The model under review builds one solid part; all positions refer to its coordinate system, in mm. Face numbers are marked on the shaded views. A direction names the side the tool comes from. Round coordinates to 2 decimals unless told otherwise and drop trailing zeros. Order: outer loops, then holes, each group sorted by start corner. A loop starts at its lowest first (then second) coordinate and runs counter-clockwise, first axis right, second up. Notation, with made-up numbers: M 48.5,-13 L 104.5,-13 A29 ccw 104.5,22 Z; hole C 23,22.5 d11. An arc over 180 degrees is marked long. Use a Markdown table: item, result. Add a question column.
1. Consider section D-D on z = -39. State the section outline as (x, y) points.
2. Insertion check: P1, Ø3, axis at x = -26.5, y = 2, coming from the -Z side; P2, Ø4, axis at y = 1.5, z = -83, coming from the -X side; P3, Ø0.8, axis at y = 7, z = -1.5, coming from the -X side; P4, Ø1, axis at x = -2.5, y = 6.5, coming from the -Z side. Each pin has a flat end and moves straight along its axis. Give the tip position at first contact, or say it passes through.
3. Consider section B-B on x = -35.5. State the section outline as (y, z) points, then the cut area to 3 significant figures.
4. For the marked faces 1 and 2, list the 3-axis set-ups (+Z, -Z, +X, -X, +Y, -Y) from which the entire face can be reached by the end or side of a thin tool; tool diameter is ignored.
5. Consider section A-A on z = -6.5. State the section outline as (x, y) points.
6. To check wall thickness, follow probe 1 along X at (y, z) = (4.25, -30); probe 2 along Z at (x, y) = (6, 8.5); probe 3 along Y at (x, z) = (26.5, -9.5). State the ranges of each line that lie inside material, in increasing order.
7. Consider section C-C on y = 7.25. Count the separate pieces of the cut face and the enclosed holes in it, then the cut area to 3 significant figures.
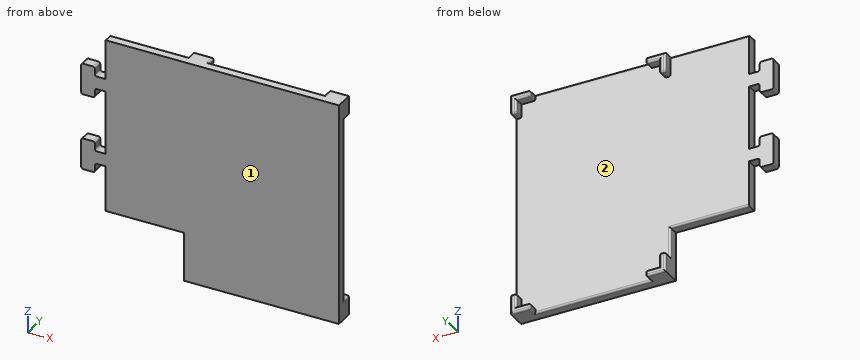
from build123d import *

# Parameters (mm, degrees)
SKETCH1_W           = 79
SKETCH1_H           = 114
BOSS_EXTRUDE1_DEPTH = 5
BOSS_EXTRUDE2_DEPTH = 5
FILLET1_R           = 1
SKETCH3_W           = 89
SKETCH3_H           = 5
BOSS_EXTRUDE3_DEPTH = 40
SKETCH4_W           = 5.5
SKETCH4_H           = 6.5
BOSS_EXTRUDE4_DEPTH = 5
FILLET2_R           = 1
FILLET3_R           = 1


with BuildPart() as part:
    # Sketch1 → Boss-Extrude1 (new body)
    with BuildSketch(Plane(origin=(0, 0, 0), x_dir=(1, 0, 0), z_dir=(0, 1, 0))):
        with Locations((39.5, 57)):
            Rectangle(SKETCH1_W, SKETCH1_H)
    extrude(amount=BOSS_EXTRUDE1_DEPTH)

    # Sketch2 → Boss-Extrude2 (add)
    with BuildSketch(Plane(origin=(0, 5, 0), x_dir=(1, 0, 0), z_dir=(0, 1, 0))):
        Polygon((0, 0), (0, 10), (3, 10), (3, 3), (10, 3), (10, 0), align=None)
        Polygon((79, 0), (69, 0), (69, 3), (76, 3), (76, 10), (79, 10), align=None)
        Polygon((79, 114), (69, 114), (69, 111), (76, 111), (76, 104), (79, 104), align=None)
        Polygon((0, 114), (0, 104), (3, 104), (3, 111), (10, 111), (10, 114), align=None)
    extrude(amount=BOSS_EXTRUDE2_DEPTH)

    # Fillet1
    fillet1_edges = [part.edges().sort_by_distance(p)[0] for p in [
        (10, 7.5, -114),
        (0, 7.5, -104),
        (3, 7.5, -104),
        (10, 7.5, -111),
        (5, 10, -114),
        (0, 10, -109),
        (1.5, 10, -104),
        (3, 10, -107.5),
        (6.5, 10, -111),
        (10, 10, -112.5),
        (79, 7.5, -104),
        (69, 7.5, -114),
        (69, 7.5, -111),
        (76, 7.5, -104),
        (79, 10, -109),
        (74, 10, -114),
        (69, 10, -112.5),
        (72.5, 10, -111),
        (76, 10, -107.5),
        (77.5, 10, -104),
        (79, 7.5, -10),
        (76, 7.5, -10),
        (69, 7.5, -3),
        (69, 7.5, 0),
        (79, 10, -5),
        (77.5, 10, -10),
        (76, 10, -6.5),
        (72.5, 10, -3),
        (69, 10, -1.5),
        (74, 10, 0),
        (10, 7.5, 0),
        (10, 7.5, -3),
        (3, 7.5, -10),
        (0, 7.5, -10),
        (5, 10, 0),
        (10, 10, -1.5),
        (6.5, 10, -3),
        (3, 10, -6.5),
        (1.5, 10, -10),
        (0, 10, -5),
    ]]
    fillet(fillet1_edges, radius=FILLET1_R)

    # Sketch3 → Boss-Extrude3 (add)
    with BuildSketch(Plane.ZY):
        with Locations((-44.5, 2.5)):
            Rectangle(SKETCH3_W, SKETCH3_H)
    extrude(amount=BOSS_EXTRUDE3_DEPTH)

    # Sketch4 → Boss-Extrude4 (add)
    with BuildSketch(Plane(origin=(0, 5, 0), x_dir=(1, 0, 0), z_dir=(0, 1, 0))):
        Polygon((-45.5, 15.5), (-45.5, 20.25), (-45.5, 26.75), (-45.5, 31.5), (-52.5, 31.5), (-52.5, 15.5), align=None)
        with Locations((-42.75, 23.5)):
            Rectangle(SKETCH4_W, SKETCH4_H)
        Polygon((-45.5, 54.5), (-45.5, 59.25), (-45.5, 65.75), (-45.5, 70.5), (-52.5, 70.5), (-52.5, 54.5), align=None)
        with Locations((-42.75, 62.5)):
            Rectangle(SKETCH4_W, SKETCH4_H)
    extrude(amount=-BOSS_EXTRUDE4_DEPTH)

    # Fillet2
    fillet2_edges = [part.edges().sort_by_distance(p)[0] for p in [
        (-52.5, 2.5, -31.5),
        (-45.5, 2.5, -31.5),
        (-45.5, 2.5, -26.75),
        (-45.5, 2.5, -20.25),
        (-45.5, 2.5, -15.5),
        (-52.5, 2.5, -15.5),
        (-52.5, 2.5, -70.5),
        (-45.5, 2.5, -70.5),
        (-45.5, 2.5, -65.75),
        (-45.5, 2.5, -59.25),
        (-45.5, 2.5, -54.5),
        (-52.5, 2.5, -54.5),
    ]]
    fillet(fillet2_edges, radius=FILLET2_R)

    # Fillet3
    fillet3_edges = [part.edges().sort_by_distance(p)[0] for p in [
        (-20, 5, -89),
        (0, 5, -97),
        (39.5, 5, -114),
        (79, 5, -57),
        (39.5, 5, 0),
        (-20, 5, 0),
    ]]
    fillet(fillet3_edges, radius=FILLET3_R)


solid = part.part
Answer block:
| question | item | result |
|---|---|---|
| 1 | outline | M -40,0 L 79,0 L 79,4 A1 ccw 78,5 L -40,5 Z |
| 2 | P1 | z = -89 |
| 2 | P2 | x = -40 |
| 2 | P3 | x = 0 |
| 2 | P4 | through |
| 3 | outline | M 0,-89 L 4,-89 A1 ccw 5,-88 L 5,-1 A1 ccw 4,0 L 0,0 Z |
| 3 | area | 445 mm^2 |
| 4 | face 1 | +Z, -Z, +X, -X, -Y |
| 4 | face 2 | +Y |
| 5 | outline | M -40,0 L 79,0 L 79,9 A1 ccw 78,10 L 77,10 A1 ccw 76,9 L 76,5 L 3,5 L 3,9 A1 ccw 2,10 L 1,10 A1 ccw 0,9 L 0,5 L -40,5 Z |
| 6 | probe 1 | -52.5 to -45.5, -40 to 78.97 |
| 6 | probe 2 | -114 to -111, -3 to 0 |
| 6 | probe 3 | 0 to 5 |
| 7 | separate pieces | 4 |
| 7 | enclosed holes | 0 |
| 7 | area | 201 mm^2 |
